Source: CAD feature listing. Evaluate the final solid. Frame: model axes, mm. A direction names the side the tool comes from. Give positions to 0.01 mm unless a question says otherwise; leave off trailing zeros. Write each loop counter-clockwise with the first axis right and the second up, starting at its lowest first coordinate (ties: lowest second). Pieces come first, ordered by that corner, then holes. Notation, with made-up numbers: (65.5, 80) -> (77.5, 80) arc R33 cw to (77.5, 117) -> close; hole circle Ø4 at (57, 48.5). An arc over 180 degrees is marked (long way). Write item = value, one per line.
from build123d import *

# Parameters (mm, degrees)
CUT_EXTRUDE1_DEPTH      = 12.340751562
CUT_EXTRUDE1_DEPTH_BACK = 12.340751562
SKETCH3_R               = 1.1938
FILLET1_R               = 0.1190625


with BuildPart() as part:
    # Sketch2 → Revolve1 (revolve)
    with BuildSketch(Plane(origin=(0, 0, 0), x_dir=(0, 0, -1), z_dir=(1, 0, 0)), mode=Mode.PRIVATE) as revolve1_sk:
        Polygon((10.25525, 1.5875), (-8.636, 1.5875), (-8.636, 3.175), (-10.175875, 3.175), (-10.414, 2.936875), (-10.414, 0), (10.414, 0), (10.414, 1.42875), align=None)
    revolve(revolve1_sk.sketch.rotate(Axis((0, 0, 10.414), (0, 0, -1)), 90), axis=Axis((0, 0, 10.414), (0, 0, -1)))

    # Sketch3 → Cut-Extrude1 (cut, two sides: drawn at the far end of the back side and taken through both)
    with BuildSketch(Plane(origin=(0, 0, 0), x_dir=(0, 0, -1), z_dir=(1, 0, 0)).offset(-CUT_EXTRUDE1_DEPTH_BACK)):
        with Locations((8.0264, 0)):
            Circle(SKETCH3_R)
    extrude(amount=CUT_EXTRUDE1_DEPTH + CUT_EXTRUDE1_DEPTH_BACK, mode=Mode.SUBTRACT)

    # Fillet1
    fillet1_edges = [part.edges().sort_by_distance(p)[0] for p in [
        (-1.5875, 0, 8.636),
    ]]
    fillet(fillet1_edges, radius=FILLET1_R)

    # Sketch4 → Cut-Revolve1 (revolve, cut)
    with BuildSketch(Plane(origin=(0, 0, 0), x_dir=(1, 0, 0), z_dir=(0, 1, 0)), mode=Mode.PRIVATE) as cut_revolve1_sk:
        Polygon((-1.5875, 9.37895), (-1.27, 9.06145), (-1.5875, 9.06145), align=None)
        Polygon((1.5875, 9.06145), (1.5875, 9.37895), (1.27, 9.06145), align=None)
    revolve(cut_revolve1_sk.sketch.rotate(Axis((0, 0, -8.0264), (-1, 0, 0)), 324.574716417), axis=Axis((0, 0, -8.0264), (-1, 0, 0)), mode=Mode.SUBTRACT)


solid = part.part
(1) Section query D-D (z = -7.25). Return loops of the section in (x, y) (1 decimal), plus the area to 3 significant figures.
Values follow:
outline = (-1.3, -0.9) arc R1.6 ccw to (1.3, -0.9) -> close; (-1.3, 0.9) -> (1.3, 0.9) arc R1.6 ccw to start
area = 2.49 mm2
(2) Pull-direction query (Y, two-part tool) for faces 3 (the face through (-0.02, 0.052, -6.834)), 4 (the face through (0, 0, -10.414)), 5 (the face through (-1.586, -0.07, -0.738)); classes: pulls with the +Y half, pulls with the -Y half, needs draft (parallel to the pull), parting line crosses it, or undercut.
Values follow:
face_3 = undercut
face_4 = needs draft
face_5 = parting line crosses it
(3) Section query C-C (z = 5.75). Return loops of the section in (x, y) (1 decimal), plus the area to 3 significant figures.
Values follow:
outline = circle Ø3.2 at (0, 0)
area = 7.92 mm2
(4) First-contact query: pin 1 (3 mm diameter, centred on y = 0, z = -8.03, fed in from -X); pin 2 (2 mm diameter, centred on x = 1, z = 1, fed in from -Y); pin 3 (1.9 mm diameter, centred on x = 1.5, y = 1.5, fed in from -Z). Flat tips, straight axial feed; report the tip coordinate or a pass-through.
Values follow:
pin_1 = -1.59
pin_2 = -1.59
pin_3 = -10.41
(5) Access query for faces 1 (the face through (-1.4, 1.4, 8.636)), 2 (the face through (-2.52, 1.93, 9.42)). Directions: +Z, -Z, +X, -X, +Y, -Y. A direction counts if a zero-diameter tool reaches every point of the face in a straight line with its end or side. Return the directions, or none.
Values follow:
face_1 = -Z
face_2 = +Z, -Z
(6) Material intervals for line 1 (Z direction, x = 0.4, y = 0); line 2 (Z direction, x = 0.75, y = 2.25); line 3 (Z direction, x = -0.5, y = 0.25), sorted ascending.
Values follow:
line_1 = -10.41 to -9.22, -6.83 to 10.41
line_2 = 8.64 to 10.41
line_3 = -10.41 to -9.19, -6.86 to 10.41
